Here's the drawing with two shaded views (mm, measured from the low corner). I have some questions. A direction names the side the tool comes from. Coordinates: 2 decimals unless noted, no trailing zeros. Order: outer loops, then holes, each group sorted by start corner. A loop starts at its lowest first (then second) coordinate and runs counter-clockwise, first axis right, second up. Notation, with made-up numbers: (23.25, -13) -> (67.25, -13) arc R28 cw to (67.25, 8) -> close; hole circle Ø10 at (13.5, -16). An arc over 180 degrees is marked (long way). Answer as a JSON object with one key per item and string values. Group by question number.
(1) I need wall thicknesses on line 1 (X direction, y = 15.75, z = 22); line 2 (Y direction, x = 7.5, z = 42); line 3 (X direction, y = 6.75, z = 22). Which ranges of each line are inside material? Lowest first, please.
(2) If we mould it in two halves opening along X, with no side actions, what happens to the marked faces 4, 5 and 6? For each: pulls with the +X half, pulls with the -X half, needs draft (parallel to the pull), parting line crosses it, or undercut.
(3) I want a section at C-C, the plane z = 31.5. List the corners of the cut face in (x, y) for me.
(4) For pin 1 (4 mm diameter, centred on x = 3, y = 19, fed in from +Z); pin 2 (6 mm diameter, centred on y = 20, z = 28, fed in from -X); pin 3 (10 mm diameter, centred on x = 7.5, y = 5.5, fed in from -Z); pin 4 (1.5 mm diameter, centred on x = 12.5, y = 8, fed in from +Z), each with a flat end and sliding along its axis, tell me the tip position at first contact or that it passes through.
(5) I want a section at D-D, the plane x = 10. State how many separate pieces and enclosed holes the cut face has, plus the area to 3 significant figures.
(6) I want a section at A-A, the plane z = 22. List the corners of the cut face in (x, y) for me.
(7) I want a section at B-B, the plane y = 14. List the corners of the cut face in (x, z) for me.
(8) Which directions (+Z, -Z, +X, -X, +Y, -Y) give clear straight access to the entire face, cutting with the end or side of a thin tool? Please do the marked faces 1, 2 and 3.
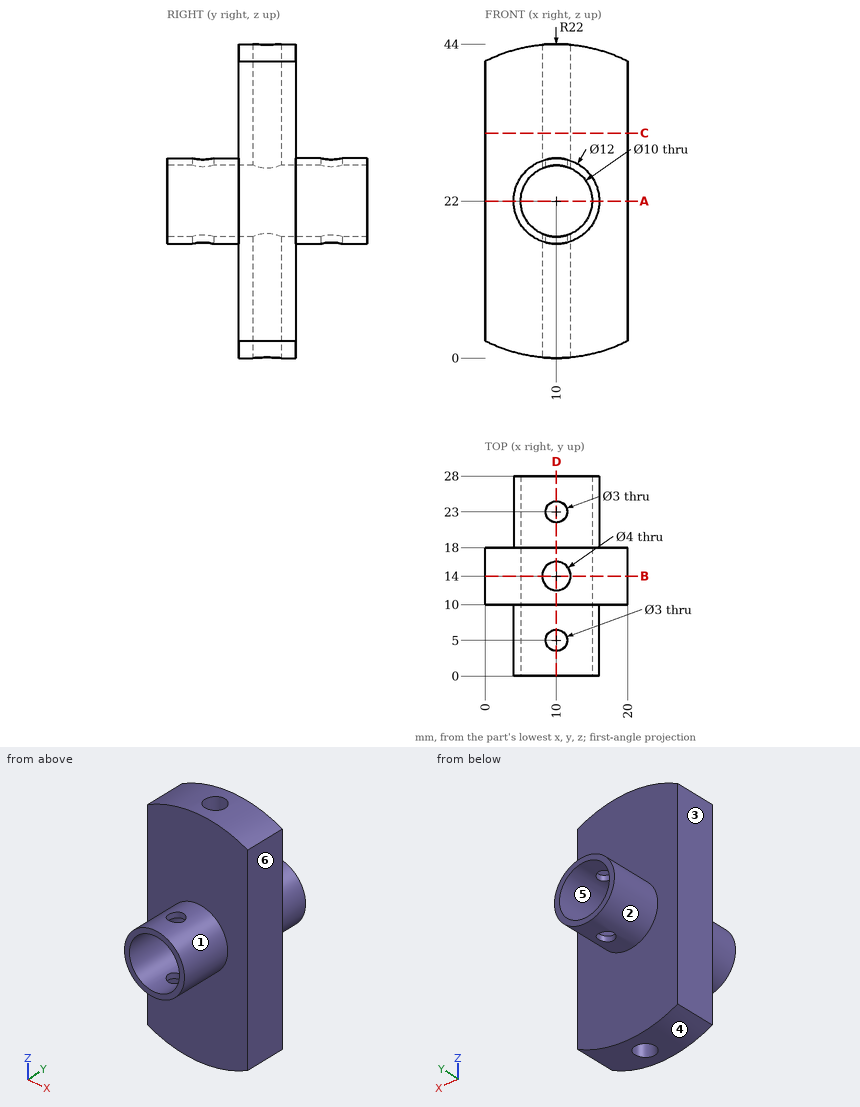
Computed values:
{
 "1": {"line 1": "x = 0 to 5, 15 to 20", "line 2": "y = 10 to 18", "line 3": "x = 4 to 5, 15 to 16"},
 "2": {"face 4": "parting line crosses it", "face 5": "undercut", "face 6": "pulls with the +X half"},
 "3": {"outline": "(0, 10) -> (20, 10) -> (20, 18) -> (0, 18) -> close; hole circle Ø4 at (10, 14)"},
 "4": {"pin 1": "stops at z = 43.36", "pin 2": "stops at x = 0", "pin 3": "stops at z = 0", "pin 4": "stops at z = 27.74"},
 "5": {"separate pieces": "8", "enclosed holes": "0", "area": "164 mm2"},
 "6": {"outline": "(0, 10) -> (4, 10) -> (4, 0) -> (5, 0) -> (5, 28) -> (4, 28) -> (4, 18) -> (0, 18) -> close; (15, 0) -> (16, 0) -> (16, 10) -> (20, 10) -> (20, 18) -> (16, 18) -> (16, 28) -> (15, 28) -> close"},
 "7": {"outline": "(0, 2.4) arc R22 ccw to (8, 0.09) -> (8, 17.42) arc R5 cw to (8, 26.58) -> (8, 43.91) arc R22 ccw to (0, 41.6) -> close; (12, 0.09) arc R22 ccw to (20, 2.4) -> (20, 41.6) arc R22 ccw to (12, 43.91) -> (12, 26.58) arc R5 cw to (12, 17.42) -> close"},
 "8": {"face 1": "-Y", "face 2": "+Y", "face 3": "+Z, -Z, -X, +Y, -Y"}
}
